```python
from build123d import *

# Parameters (mm, degrees)
CROQUIS1_W              = 111
CROQUIS1_H              = 94
CROQUIS1_W_2            = 10
CROQUIS1_H_2            = 3
SALIENTE_EXTRUIR1_DEPTH = 3


with BuildPart() as part:
    # Croquis1 → Saliente-Extruir1 (new body)
    with BuildSketch(Plane(origin=(0, 0, 0), x_dir=(1, 0, 0), z_dir=(0, 1, 0))):
        with Locations((48.5, 40)):
            Rectangle(CROQUIS1_W, CROQUIS1_H)
        with BuildLine():
            Line((7, 0), (0, 0))
            Line((0, 0), (0, 25.625))
            Line((0, 25.625), (-1.5, 25.625))
            ThreePointArc((-1.5, 25.625), (-2.875, 27), (-1.5, 28.375))
            Line((-1.5, 28.375), (0, 28.375))
            Line((0, 28.375), (0, 51.625))
            Line((0, 51.625), (-1.5, 51.625))
            ThreePointArc((-1.5, 51.625), (-2.875, 53), (-1.5, 54.375))
            Line((-1.5, 54.375), (0, 54.375))
            Line((0, 54.375), (0, 80))
            Line((0, 80), (7, 80))
            Line((7, 80), (7, 83))
            Line((7, 83), (17, 83))
            Line((17, 83), (17, 80))
            Line((17, 80), (30.775145502, 80))
            Line((30.775145502, 80), (30.775000006, 81.499866617))
            ThreePointArc((30.775000006, 81.499866617), (32.149933309, 82.874999998), (33.525, 81.5))
            Line((33.525, 81.5), (33.525, 80))
            Line((33.525, 80), (63.475, 80))
            Line((63.475, 80), (63.475, 81.500066988))
            ThreePointArc((63.475, 81.500066988), (64.850028215, 82.875038772), (66.225, 81.500010557))
            Line((66.225, 81.500010557), (66.225, 80))
            Line((66.225, 80), (66.475145502, 80))
            Line((66.475145502, 80), (74.57, 80))
            Line((74.57, 80), (74.57, 65))
            Line((74.57, 65), (77.57, 65))
            Line((77.57, 65), (77.57, 55))
            Line((77.57, 55), (74.57, 55))
            Line((74.57, 55), (74.57, 25))
            Line((74.57, 25), (77.57, 25))
            Line((77.57, 25), (77.57, 15))
            Line((77.57, 15), (74.57, 15))
            Line((74.57, 15), (74.57, 0))
            Line((74.57, 0), (66.225, 0))
            Line((66.225, 0), (66.225, -1.500010557))
            ThreePointArc((66.225, -1.500010557), (64.850028215, -2.875038772), (63.475, -1.500066988))
            Line((63.475, -1.500066988), (63.475, 0))
            Line((63.475, 0), (33.525, 0))
            Line((33.525, 0), (33.525, -1.5))
            ThreePointArc((33.525, -1.5), (32.149933309, -2.874999998), (30.775000006, -1.499866617))
            Line((30.775000006, -1.499866617), (30.775145502, 0))
            Line((30.775145502, 0), (17, 0))
            Line((17, 0), (17, -3))
            Line((17, -3), (7, -3))
            Line((7, -3), (7, 0))
        make_face(mode=Mode.SUBTRACT)
        with Locations((85, -1.5)):
            Rectangle(CROQUIS1_W_2, CROQUIS1_H_2, mode=Mode.SUBTRACT)
        with BuildLine():
            ThreePointArc((98.5, 28.375), (99.875, 27), (98.5, 25.625))
            Line((98.5, 25.625), (95.5, 25.625))
            ThreePointArc((95.5, 25.625), (94.125, 27), (95.5, 28.375))
            Line((95.5, 28.375), (98.5, 28.375))
        make_face(mode=Mode.SUBTRACT)
        with BuildLine():
            ThreePointArc((98.5, 54.375), (99.875, 53), (98.5, 51.625))
            Line((98.5, 51.625), (95.5, 51.625))
            ThreePointArc((95.5, 51.625), (94.125, 53), (95.5, 54.375))
            Line((95.5, 54.375), (98.5, 54.375))
        make_face(mode=Mode.SUBTRACT)
        with Locations((85, 81.5)):
            Rectangle(CROQUIS1_W_2, CROQUIS1_H_2, mode=Mode.SUBTRACT)
    extrude(amount=SALIENTE_EXTRUIR1_DEPTH)


solid = part.part
```
Here's how the part is built. I have some questions about the finished solid (model axes, mm). A direction names the side the tool comes from. Coordinates: 2 decimals unless noted, no trailing zeros. Write each loop counter-clockwise with the first axis right and the second up, starting at its lowest first coordinate (ties: lowest second). Pieces come first, ordered by that corner, then holes. Notation, with made-up numbers: (20, 62.5) - (48, 62.5) arc R34 ccw to (48, 99.5) - close; hole circle Ø3 at (-14, 22.5). An arc over 180 degrees is marked (long way). One line per item, written item: value.
1) Suppose I cut it at C-C on x = 85. Write out the boundary of the cut face in (y, z).
Model answer:
outline: (0, -87) - (3, -87) - (3, -83) - (0, -83) - close; (0, -80) - (3, -80) - (3, 0) - (0, 0) - close; (0, 3) - (3, 3) - (3, 7) - (0, 7) - close
2) Suppose I cut it at B-B on z = -27. Write out the boundary of the cut face in (x, y) (3 decimals), and give its area (3 significant figures).
Model answer:
outline: (-7, 0) - (-2.875, 0) - (-2.875, 3) - (-7, 3) - close; (74.57, 0) - (94.125, 0) - (94.125, 3) - (74.57, 3) - close; (99.875, 0) - (104, 0) - (104, 3) - (99.875, 3) - close
area: 83.4 mm²
3) I need wall thicknesses on line 1 along Z through (x, y) = (89.5, 1.8); line 2 along Z through (x, y) = (-1, 2.5) (3 decimals); line 3 along X through (y, z) = (0.65, -34). Which ranges of each line are inside material? Lowest first, please.
Model answer:
line 1: z = -87 to -83, -80 to 0, 3 to 7
line 2: z = -87 to -54.375, -51.625 to -28.375, -25.625 to 7
line 3: x = -7 to 0, 74.57 to 104
4) Suppose I cut it at D-D on z = -58. Write out the boundary of the cut face in (x, y), and give its area (3 significant figures).
Model answer:
outline: (-7, 0) - (0, 0) - (0, 3) - (-7, 3) - close; (77.57, 0) - (104, 0) - (104, 3) - (77.57, 3) - close
area: 100 mm²
5) On a 3-axis mill with a long thin cutter (end or side, diameter ignored), from which of +Z, -Z, +X, -X, +Y, -Y can I reach the whole of each face in a straight line? I mean faces 1 (the flat face through (17, 1, -82)), 2 (the flat face through (85, 0, -41)). Say none if no direction works.
Model answer:
face 1: +Y, -Y
face 2: +Z, -Z, +X, -X, -Y
6) I'm going to push a flat-ended pin straight in: P1, Ø1.5, axis at x = 87, z = -62, coming from the -Y side. Where does the tip first touch, or does it pass through?
Model answer:
P1: stops at y = 0
7) Suppose I cut it at A-A on x = 64.85. Write out the boundary of the cut face in (y, z), and give its area (3 significant figures).
Model answer:
outline: (0, -87) - (3, -87) - (3, -82.88) - (0, -82.88) - close; (0, 2.88) - (3, 2.88) - (3, 7) - (0, 7) - close
area: 24.7 mm²
8) We'd pull the mould along Z, two halves only. Please class faces 3 (the flat face through (7, 1, -81)), 4 (the flat face through (85, 3, -41)), 5 (the cylindrical face through (-2.875, 1.479, -52.97)): pulls with the +Z half, pulls with the -Z half, needs draft (parallel to the pull), parting line crosses it, or undercut.
Model answer:
face 3: undercut
face 4: needs draft
face 5: undercut
